Can you work these out from the model? Positions are in its coordinate system, mm. A direction names the side the tool comes from. Coordinates: 2 decimals unless noted, no trailing zeros. Write each loop counter-clockwise with the first axis right and the second up, starting at its lowest first coordinate (ties: lowest second). Pieces come first, ordered by that corner, then holes. Notation, with made-up numbers: (47, -12) - (91, -12) arc R14 cw to (91, 9) - close; hole circle Ø3 at (-30.75, -23). An arc over 180 degrees is marked (long way). Use one line per item in the form item = value. Start each with the question number.
(1) If we section it at B-B on z = -18: Please give me the cut outline in (x, y).
(2) For pin 1 Ø2.5 at (x, z) = (13, -36.5) entering from -Y; pin 2 Ø2.5 at (x, z) = (14, -36) entering from +Y; pin 3 Ø5.5 at (y, z) = (-1, 4) entering from -X; pin 4 Ø3 at (y, z) = (-33, 22.5) entering from +X, each with a flat end and sliding along its axis, tell me the tip position at first contact or that it passes through.
(3) On a 3-axis mill with a long thin cutter (end or side, diameter ignored), from which of +Z, -Z, +X, -X, +Y, -Y can I reach the whole of each face in a straight line? I mean faces 1 (the face through (6, 0, -42.789)), 2 (the face through (7, 28.969, 33)), 3 (the face through (13, 0, 19.054)). Say none if no direction works.
(4) If we section it at C-C on y = -27: Please give me the cut outline in (x, z), then the cut area to 3 significant figures.
(5) If I drill on probe 1 along Y at (x, z) = (8.25, -2.5); probe 2 along Y at (x, z) = (6.75, -25); probe 3 along X at (y, z) = (9, 33), over which ranges is the centre line in solid material (lowest first)? Write a range as from..to.
(6) If we section it at D-D on z = 23: Please give me the cut outline in (x, y).
(7) Thinking about a two-plate mould opening in Z: for faces 4 (the face through (7.4, 26, -39.9)), 5 (the face through (13.52, 10.5, 23.69)), 6 (the face through (12.5, -4, 2)), 7 (the face through (7, -28.969, 33)), which applies, pulls with the +Z half, pulls with the -Z half, needs draft (parallel to the pull), parting line crosses it, or undercut?
(8) If we section it at A-A on x = 4.5: Please give me the cut outline in (y, z), then the cut area to 3 significant figures.
```python
from build123d import *

# Parameters (mm, degrees)
BOSS_EXTRUDE3_DEPTH = 15
SKETCH3_R           = 4
CUT_EXTRUDE3_DEPTH  = 14.0462
CUT_EXTRUDE4_DEPTH  = 3
CUT_EXTRUDE5_START  = -15
CUT_EXTRUDE5_DEPTH  = 12.5
MIRROR1_DEPTH       = 12.5
MIRROR1_START       = 12
MIRROR1_2_DEPTH     = 3
MIRROR1_3_DEPTH     = 12
MIRROR1_4_DEPTH     = 3


# Read off the part's stored shape, not the designer's step: Mirror1
with BuildPart() as part:
    # Sketch1 → Boss-Extrude3 (new body)
    with BuildSketch(Plane.YZ):
        with BuildLine():
            Line((-28.968617751, -12.789334175), (28.968617751, -12.789334175))
            ThreePointArc((28.968617751, -12.789334175), (44.579120821, 0), (35.110840206, 17.821518929))
            ThreePointArc((35.110840206, 17.821518929), (30.644623053, 21.505675602), (28.968617751, 27.047436358))
            Line((28.968617751, 27.047436358), (28.968617751, 39.053986921))
            ThreePointArc((28.968617751, 39.053986921), (26.039685563, 46.125054733), (18.968617751, 49.053986921))
            Line((18.968617751, 49.053986921), (-18.968617751, 49.053986921))
            ThreePointArc((-18.968617751, 49.053986921), (-26.039685563, 46.125054733), (-28.968617751, 39.053986921))
            Line((-28.968617751, 39.053986921), (-28.968617751, 27.047436358))
            ThreePointArc((-28.968617751, 27.047436358), (-30.644623053, 21.505675602), (-35.110840206, 17.821518929))
            ThreePointArc((-35.110840206, 17.821518929), (-44.579120821, 0), (-28.968617751, -12.789334175))
        make_face()
    extrude(amount=BOSS_EXTRUDE3_DEPTH)

    # Sketch3 → Cut-Extrude3 (cut)
    with BuildSketch(Plane.YZ.offset(15)):
        with Locations(Location((0, 3.132326373, 0), (0, 0, 270))):
            Circle(SKETCH3_R)
    extrude(amount=-CUT_EXTRUDE3_DEPTH, mode=Mode.SUBTRACT)

    # Sketch4 → Cut-Extrude4 (cut)
    with BuildSketch(Plane.YZ.offset(15)):
        with BuildLine():
            Line((-12.95, 49.053986921), (-12.95, 31.267703884))
            ThreePointArc((-12.95, 31.267703884), (0, 18.317703884), (12.95, 31.267703884))
            Line((12.95, 31.267703884), (12.95, 49.053986921))
            Line((12.95, 49.053986921), (-12.95, 49.053986921))
        make_face()
    extrude(amount=-CUT_EXTRUDE4_DEPTH, mode=Mode.SUBTRACT)

    # Sketch5 → Cut-Extrude5 (cut, symmetric)
    with BuildSketch(Plane.YZ.offset(15).offset(CUT_EXTRUDE5_START)):
        Polygon((5.466157569, 6.586954394), (-0.258716842, 9.5934717), (-5.724874411, 6.138843679), (-5.466157569, -0.322301647), (0.258716842, -3.328818953), (5.724874411, 0.125809067), align=None)
    extrude(amount=CUT_EXTRUDE5_DEPTH, both=True, mode=Mode.SUBTRACT)

    # Mirror1 outline → Mirror1 (cut)
    with BuildSketch(Plane.YZ):
        Polygon((-2.802243807, -1.721302263), (-0.258716842, -3.328818953), (0, -3.192949306), align=None)
        Polygon((-5.724874411, 0.125809067), (-5.477849424, -0.030311467), (-5.604487603, 3.132326373), align=None)
        Polygon((5.477849424, -0.030311467), (2.802243807, -1.721302263), (5.466157569, -0.322301647), align=None)
        Polygon((-5.466157569, 6.586954394), (-5.477849424, 6.294964213), (-2.802243802, 7.985955012), align=None)
        Polygon((5.477849424, 6.294964213), (5.604487603, 3.132326373), (5.724874411, 6.138843679), align=None)
        Polygon((0.258716842, 9.5934717), (0, 9.457602053), (2.802243802, 7.985955012), align=None)
    extrude(amount=MIRROR1_DEPTH, mode=Mode.SUBTRACT)

    # Mirror1 2 outline → Mirror1 2 (cut)
    with BuildSketch(Plane.YZ.offset(MIRROR1_START)):
        with BuildLine():
            ThreePointArc((4.30437196, -12.789334175), (0, -12.053051137), (-4.30437196, -12.789334175))
            Line((-4.30437196, -12.789334175), (4.30437196, -12.789334175))
        make_face()
    extrude(amount=MIRROR1_2_DEPTH, mode=Mode.SUBTRACT)

    # Mirror1 3 outline → Mirror1 3 (add)
    with BuildSketch(Plane.YZ):
        with BuildLine():
            ThreePointArc((-28.968617751, -32.789334175), (-26.039685563, -39.860401987), (-18.968617751, -42.789334175))
            Line((-18.968617751, -42.789334175), (18.968617751, -42.789334175))
            ThreePointArc((18.968617751, -42.789334175), (26.039685563, -39.860401987), (28.968617751, -32.789334175))
            Line((28.968617751, -32.789334175), (28.968617751, -20.782783611))
            ThreePointArc((28.968617751, -20.782783611), (30.644623053, -15.241022855), (35.110840206, -11.556866182))
            ThreePointArc((35.110840206, -11.556866182), (32.100944124, -12.478176697), (28.968617751, -12.789334175))
            Line((28.968617751, -12.789334175), (-28.968617751, -12.789334175))
            ThreePointArc((-28.968617751, -12.789334175), (-32.100944124, -12.478176697), (-35.110840206, -11.556866182))
            ThreePointArc((-35.110840206, -11.556866182), (-30.644623053, -15.241022855), (-28.968617751, -20.782783611))
            Line((-28.968617751, -20.782783611), (-28.968617751, -32.789334175))
        make_face()
        Polygon((-5.466157569, -0.322301647), (-2.802243807, -1.721302263), (-5.477849424, -0.030311467), align=None)
        Polygon((2.802243807, -1.721302263), (0, -3.192949306), (0.258716842, -3.328818953), align=None)
        Polygon((-5.724874411, 6.138843679), (-5.604487603, 3.132326373), (-5.477849424, 6.294964213), align=None)
        Polygon((5.604487603, 3.132326373), (5.477849424, -0.030311467), (5.724874411, 0.125809067), align=None)
        Polygon((-0.258716842, 9.5934717), (-2.802243802, 7.985955012), (0, 9.457602053), align=None)
        Polygon((2.802243802, 7.985955012), (5.477849424, 6.294964213), (5.466157569, 6.586954394), align=None)
    extrude(amount=MIRROR1_3_DEPTH)

    # Mirror1 4 outline → Mirror1 4 (add)
    with BuildSketch(Plane.YZ.offset(MIRROR1_START)):
        with BuildLine():
            ThreePointArc((-28.968617751, -32.789334175), (-26.039685563, -39.860401987), (-18.968617751, -42.789334175))
            Line((-18.968617751, -42.789334175), (-12.95, -42.789334175))
            Line((-12.95, -42.789334175), (-12.95, -25.003051137))
            ThreePointArc((-12.95, -25.003051137), (-10.569865583, -17.521043281), (-4.30437196, -12.789334175))
            Line((-4.30437196, -12.789334175), (-28.968617751, -12.789334175))
            ThreePointArc((-28.968617751, -12.789334175), (-32.100944124, -12.478176697), (-35.110840206, -11.556866182))
            ThreePointArc((-35.110840206, -11.556866182), (-30.644623053, -15.241022855), (-28.968617751, -20.782783611))
            Line((-28.968617751, -20.782783611), (-28.968617751, -32.789334175))
        make_face()
        with BuildLine():
            Line((12.95, -25.003051137), (12.95, -42.789334175))
            Line((12.95, -42.789334175), (18.968617751, -42.789334175))
            ThreePointArc((18.968617751, -42.789334175), (26.039685563, -39.860401987), (28.968617751, -32.789334175))
            Line((28.968617751, -32.789334175), (28.968617751, -20.782783611))
            ThreePointArc((28.968617751, -20.782783611), (30.644623053, -15.241022855), (35.110840206, -11.556866182))
            ThreePointArc((35.110840206, -11.556866182), (32.100944124, -12.478176697), (28.968617751, -12.789334175))
            Line((28.968617751, -12.789334175), (4.30437196, -12.789334175))
            ThreePointArc((4.30437196, -12.789334175), (10.569865583, -17.521043281), (12.95, -25.003051137))
        make_face()
        with BuildLine():
            ThreePointArc((-4.304371959, 19.053986921), (0, 18.317703884), (4.304371959, 19.053986921))
            Line((4.304371959, 19.053986921), (-4.304371959, 19.053986921))
        make_face()
        Polygon((-5.466157569, -0.322301647), (-2.802243807, -1.721302263), (-5.477849424, -0.030311467), align=None)
        Polygon((2.802243807, -1.721302263), (0, -3.192949306), (0.258716842, -3.328818953), align=None)
        Polygon((-5.724874411, 6.138843679), (-5.604487603, 3.132326373), (-5.477849424, 6.294964213), align=None)
        Polygon((5.604487603, 3.132326373), (5.477849424, -0.030311467), (5.724874411, 0.125809067), align=None)
        Polygon((-0.258716842, 9.5934717), (-2.802243802, 7.985955012), (0, 9.457602053), align=None)
        Polygon((2.802243802, 7.985955012), (5.477849424, 6.294964213), (5.466157569, 6.586954394), align=None)
    extrude(amount=MIRROR1_4_DEPTH)


solid = part.part
```
Reported:
q1.outline = (0, -29.36) - (15, -29.36) - (15, -10.89) - (12, -10.89) - (12, 10.89) - (15, 10.89) - (15, 29.36) - (0, 29.36) - close
q2.pin_1 = -28.66
q2.pin_2 = 28.77
q2.pin_3 = 12.5
q2.pin_4 = through
q3.face_1 = -Z, +X, -X, +Y, -Y
q3.face_2 = +Z, +X, -X, +Y
q3.face_3 = +Z, +X
q4.outline = (0, -38.75) - (15, -38.75) - (15, 45.01) - (0, 45.01) - close
q4.area = 1,260 mm2
q5.probe_1 = -43.86..-1.57, 1.32..43.86
q5.probe_2 = -28.97..28.97
q5.probe_3 = 0..12
q6.outline = (0, -29.82) - (15, -29.82) - (15, -9.97) - (12, -9.97) - (12, 9.97) - (15, 9.97) - (15, 29.82) - (0, 29.82) - close
q7.face_4 = pulls with the -Z half
q7.face_5 = pulls with the +Z half
q7.face_6 = undercut
q7.face_7 = needs draft
q8.outline = (-35.11, -11.56) arc R10 cw to (-28.97, -20.78) - (-28.97, -32.79) arc R10 ccw to (-18.97, -42.79) - (18.97, -42.79) arc R10 ccw to (28.97, -32.79) - (28.97, -20.78) arc R10 cw to (35.11, -11.56) arc R15.92 ccw to (35.11, 17.82) arc R10 cw to (28.97, 27.05) - (28.97, 39.05) arc R10 ccw to (18.97, 49.05) - (-18.97, 49.05) arc R10 ccw to (-28.97, 39.05) - (-28.97, 27.05) arc R10 cw to (-35.11, 17.82) arc R15.92 ccw to start; hole (-5.72, 0.13) - (-0.26, -3.33) - (5.47, -0.32) - (5.72, 6.14) - (0.26, 9.59) - (-5.47, 6.59) - close
q8.area = 5,970 mm2
